from build123d import *

# Parameters (mm, degrees)
F1_DEPTH = 50.8
F2_R     = 5.08


with BuildPart() as f1:
    # F0 (on Front) → F1 (new body)
    with BuildSketch(Plane.XZ):
        Polygon((0, 40.230382), (0, 0), (41.808043, 0), (41.808043, 22.650717), (25.355281, 22.650717), (25.355281, 40.230382), align=None)
    extrude(amount=F1_DEPTH)

    # F2
    f2_edges = [f1.edges().sort_by_distance(p)[0] for p in [
        (25.355281, -25.4, 40.230382),
        (41.808043, -25.4, 22.650717),
        (41.808043, -25.4, 0),
        (0, -25.4, 40.230382),
    ]]
    fillet(f2_edges, radius=F2_R)


solid = f1.part
Design review of the part built by this model. Coordinates are the model's own, in mm. A direction names the side the tool comes from. Round coordinates to 2 decimals unless told otherwise and drop trailing zeros. Write each loop counter-clockwise with the first axis right and the second up, starting at its lowest first coordinate (ties: lowest second). Pieces come first, ordered by that corner, then holes.
Item 1: Wall thickness on L1, parallel to X at y = -16.5, z = 34; L2, parallel to Z at x = 33, y = -18; L3, parallel to X at y = -42, z = 20.5: over which ranges is each line inside the solid? List them lowest first.
Item 2: Consider section B-B on x = 35. Give the boundary of the cut face in (y, z), and give its area (3 significant figures).
Item 3: Consider section A-A on y = -36.5. Give the boundary of the cut face in (x, z), and give its area (3 significant figures).
Item 4: For faces 1 (the cylindrical face through (1.449, -25.756, 38.703)), 2 (the flat face through (31, -25, 22.651)), list the 3-axis set-ups (+Z, -Z, +X, -X, +Y, -Y) from which the entire face can be reached by the end or side of a thin tool; tool diameter is ignored.
Item 5: Consider section C-C on x = 24. Give the boundary of the cut face in (y, z).
Item 6: For pin 1 Ø10 at (y, z) = (-26, 29.5) entering from +X; pin 2 Ø5.5 at (x, y) = (31, -31.5) entering from +Z, all flat-tipped, find the tip position at first contact; note any pin that passes through.
Check values:
1. L1: x = 0 to 25.36
1. L2: z = 0 to 22.65
1. L3: x = 0 to 40.88
2. outline: (-50.8, 0) - (0, 0) - (0, 22.65) - (-50.8, 22.65) - close
2. area: 1,150 mm2
3. outline: (0, 0) - (36.73, 0) arc R5.08 ccw to (41.81, 5.08) - (41.81, 17.57) arc R5.08 ccw to (36.73, 22.65) - (25.36, 22.65) - (25.36, 35.15) arc R5.08 ccw to (20.28, 40.23) - (5.08, 40.23) arc R5.08 ccw to (0, 35.15) - close
3. area: 1,370 mm2
4. face 1: +Z, -X, +Y, -Y
4. face 2: +Z, +X, +Y, -Y
5. outline: (-50.8, 0) - (0, 0) - (0, 38.6) - (-50.8, 38.6) - close
6. pin 1: stops at x = 25.36
6. pin 2: stops at z = 22.65
